For this review, take the finished solid that the model builds, in its own axes (mm). A direction names the side the tool comes from. Coordinates: 2 decimals unless noted, no trailing zeros. Loops run counter-clockwise (first coordinate to the right, second up) from the corner with the lowest first, then second, coordinate; pieces in that order, holes last. Notation, with made-up numbers: M 37,-38 L 41,-38 A20 cw 41,-19 Z; hole C 6.5,89 d11. An arc over 180 degrees is marked long. Use one line per item in the form item = value.
```python
from build123d import *

# Parameters (mm, degrees)
SKETCH1_W           = 22.5
SKETCH1_H           = 33
SKETCH1_W_2         = 12.5
SKETCH1_H_2         = 23
BOSS_EXTRUDE1_DEPTH = 8
SKETCH2_R           = 1.1
CUT_EXTRUDE1_DEPTH  = 22.513077418
SKETCH4_W           = 22.5
SKETCH4_H           = 12
BOSS_EXTRUDE3_DEPTH = 8
SKETCH5_W           = 22.5
SKETCH5_H           = 5
BOSS_EXTRUDE4_DEPTH = 45
SKETCH6_W           = 12.5
SKETCH6_H           = 25
CUT_EXTRUDE2_DEPTH  = 71.431260815
SKETCH7_R           = 1.1
CUT_EXTRUDE3_DEPTH  = 65
FILLET1_R           = 5
SKETCH9_W           = 22.5
SKETCH9_H           = 44.865556073
BOSS_EXTRUDE5_DEPTH = 5
SKETCH10_R          = 8.736478528
CUT_EXTRUDE4_DEPTH  = 3
FILLET2_R           = 5
FILLET3_R           = 5
FILLET4_R           = 5


with BuildPart() as part:
    # Sketch1 → Boss-Extrude1 (new body)
    with BuildSketch(Plane.XY):
        Rectangle(SKETCH1_W, SKETCH1_H)
        Rectangle(SKETCH1_W_2, SKETCH1_H_2, mode=Mode.SUBTRACT)
    extrude(amount=BOSS_EXTRUDE1_DEPTH)

    # Sketch2 → Cut-Extrude1 (cut, through all)
    with BuildSketch(Plane.XY.offset(8)):
        with Locations((0, -14.145204103)):
            Circle(SKETCH2_R)
        with Locations((0, 14.145204103)):
            Circle(SKETCH2_R)
    extrude(amount=-CUT_EXTRUDE1_DEPTH, mode=Mode.SUBTRACT)

    # Sketch4 → Boss-Extrude3 (add)
    with BuildSketch(Plane(origin=(0, 0, 0), x_dir=(-1, 0, 0), z_dir=(0, 0, -1))):
        with Locations((0, -22.5)):
            Rectangle(SKETCH4_W, SKETCH4_H)
    extrude(amount=-BOSS_EXTRUDE3_DEPTH)

    # Sketch5 → Boss-Extrude4 (add)
    with BuildSketch(Plane.XY.offset(8)):
        with Locations((0, -26)):
            Rectangle(SKETCH5_W, SKETCH5_H)
    extrude(amount=BOSS_EXTRUDE4_DEPTH)

    # Sketch6 → Cut-Extrude2 (cut, through all)
    with BuildSketch(Plane.XZ.offset(28.5)):
        with Locations((0, 26.5)):
            Rectangle(SKETCH6_W, SKETCH6_H)
    extrude(amount=-CUT_EXTRUDE2_DEPTH, mode=Mode.SUBTRACT)

    # Sketch7 → Cut-Extrude3 (cut)
    with BuildSketch(Plane.XZ.offset(28.5)):
        with Locations(Location((0, 40.645204103, 0), (0, 0, 270))):
            Circle(SKETCH7_R)
        with Locations(Location((0, 12.354795897, 0), (0, 0, 270))):
            Circle(SKETCH7_R)
    extrude(amount=-CUT_EXTRUDE3_DEPTH, mode=Mode.SUBTRACT)

    # Fillet1
    # the kernel refuses this fillet: 5 mm, written as the material it adds along each edge
    with BuildSketch(Plane(origin=(11.25, -23.5, 8), x_dir=(0, 1, 0), z_dir=(-1, 0, 0))) as fillet1_piece_1_section:
        with BuildLine():
            CenterArc((FILLET1_R, -FILLET1_R), FILLET1_R, 90, 90)
            Line((0, -FILLET1_R), (0, 0))
            Line((0, 0), (FILLET1_R, 0))
        make_face()
    fillet1_piece_1 = extrude(amount=22.5, mode=Mode.PRIVATE)
    fillet1_piece_1 = fillet1_piece_1 - Plane(origin=(0, -22.363323705, 12.354795897), x_dir=(0, 0, -1), z_dir=(0, -1, 0)) * Cylinder(1.1, 65, mode=Mode.PRIVATE)
    add(fillet1_piece_1)

    # Sketch9 → Boss-Extrude5 (add)
    with BuildSketch(Plane.XY.offset(53)):
        with Locations((0, -6.067221963)):
            Rectangle(SKETCH9_W, SKETCH9_H)
    extrude(amount=-BOSS_EXTRUDE5_DEPTH)

    # Sketch10 → Cut-Extrude4 (cut)
    with BuildSketch(Plane(origin=(0, 0, 48), x_dir=(-1, 0, 0), z_dir=(0, 0, -1))):
        with Locations((0, 5)):
            Circle(SKETCH10_R)
    extrude(amount=-CUT_EXTRUDE4_DEPTH, mode=Mode.SUBTRACT)

    # Fillet2
    fillet2_edges = [part.edges().sort_by_distance(p)[0] for p in [
        (0, -23.5, 48),
    ]]
    fillet(fillet2_edges, radius=FILLET2_R)

    # Fillet3
    fillet3_edges = [part.edges().sort_by_distance(p)[0] for p in [
        (0, -28.5, 0),
        (0, -28.5, 53),
    ]]
    fillet(fillet3_edges, radius=FILLET3_R)

    # Fillet4
    fillet4_edges = [part.edges().sort_by_distance(p)[0] for p in [
        (11.25, 16.365556073, 50.5),
        (-11.25, 16.365556073, 50.5),
        (-11.25, 16.5, 4),
        (11.25, 16.5, 4),
    ]]
    fillet(fillet4_edges, radius=FILLET4_R)


solid = part.part
```
1. For pin 1 Ø7 at (x, y) = (-1.5, 5.5) entering from -Z; pin 2 Ø1.5 at (x, y) = (3, -27) entering from -Z; pin 3 Ø3.5 at (x, z) = (0, 40.65) entering from +Y, all flat-tipped, find the tip position at first contact; note any pin that passes through.
Computed values:
pin_1 = 51
pin_2 = 0.82
pin_3 = -23.5
2. Consider section C-C on x = 0. State how many separate pieces and enclosed holes the cut face has, plus the area to 3 significant figures.
Computed values:
separate_pieces = 7
enclosed_holes = 0
area = 366 mm2
3. Consider section D-D on y = -6. Write out the cut boundary in (x, z).
Computed values:
outline = M -11.25,0 L -6.25,0 L -6.25,8 L -11.25,8 Z; M -11.25,48 L 11.25,48 L 11.25,53 L -11.25,53 Z; M 6.25,0 L 11.25,0 L 11.25,8 L 6.25,8 Z
4. Tool access review of faces 1 (the face through (-4.697, 12.367, 49.479)), 2 (the face through (0, -11.5, 4)), 3 (the face through (0, -26, 14)), 4 (the face through (9.824, 14.862, 50.465)), 5 (the face through (-7, -1, 8)): name each direction out of +Z, -Z, +X, -X, +Y, -Y from which nothing blocks a thin tool from reaching the whole face with its end or side.
Computed values:
face_1 = none
face_2 = -Z
face_3 = +Y, -Y
face_4 = +Z, +X, +Y
face_5 = +X, -X, +Y
5. Wall thickness on line 1 along Z through (x, y) = (7, 7); line 2 along Y through (x, z) = (0, 4.75); line 3 along Z through (x, y) = (9.5, -10): over which ranges is each line inside the solid? List them lowest first. Write a range as from..to.
Computed values:
line_1 = 0..8, 51..53
line_2 = -28.49..-15.25, -13.05..-11.5, 11.5..13.05, 15.25..16.5
line_3 = 0..8, 48..53
6. Consider section B-B on z = 20.5. Write out the cut boundary in (x, y).
Computed values:
outline = M -11.25,-28.5 L -6.25,-28.5 L -6.25,-23.5 L -11.25,-23.5 Z; M 6.25,-28.5 L 11.25,-28.5 L 11.25,-23.5 L 6.25,-23.5 Z
7. Draft analysis for pull direction Y (two halves, no side actions). For faces 6 (the face through (0.16, -22.07, 46.5)), 7 (the face through (0.51, -15.12, 4.06)), 8 (the face through (0, -5, 48)), state which applies: +Y half, -Y half, draft (parallel to the pull), parting line (faces both ways), or undercut.
Computed values:
face_6 = +Y half
face_7 = undercut
face_8 = draft
8. Consider section A-A on y = 5. Write out the cut boundary in (x, z), plus the area to 3 significant figures.
Computed values:
outline = M -11.25,0 L -6.25,0 L -6.25,8 L -11.25,8 Z; M -11.25,48 L -8.74,48 L -8.74,51 L 8.74,51 L 8.74,48 L 11.25,48 L 11.25,53 L -11.25,53 Z; M 6.25,0 L 11.25,0 L 11.25,8 L 6.25,8 Z
area = 140 mm2
